Answer from the drawing. Dimensions are ordinates in mm from the lowest x, y and z of the part. Coordinates: 2 decimals unless noted, no trailing zeros. Order: outer loops, then holes, each group sorted by start corner. A loop starts at its lowest first (then second) coordinate and runs counter-clockwise, first axis right, second up. Notation, with made-up numbers: (83.5, 71) -> (105.5, 71) arc R18 cw to (105.5, 85) -> close; hole circle Ø2 at (-31.5, 79). An arc over 180 degrees is marked (long way). Answer as a JSON object with one key per item and string values. Group by question number.
1) Consider L1, parallel to Y at x = 95, z = 2.3; L2, parallel to X at y = 140, z = 3.25; L3, parallel to X at y = 130, z = 2.75. Determine where each line is inside the solid, lowest interval first.
2) Section A-A on z = 2.7 is taken. Determine the outline of the cut face in (x, y), and give its area (3 significant figures).
3) Section B-B on x = 60.5 is taken. Determine the outline of the cut face in (y, z), and give its area (3 significant figures).
4) Given pin 1 (2 mm diameter, centred on x = 68, z = 3.5, fed in from -Y); pin 2 (2 mm diameter, centred on y = 180, z = 3, fed in from -X), each flat-ended and moving along its own axis, determine where each tip first touches the part or whether it passes through.
5) Section C-C on y = 154 is taken. Determine the outline of the cut face in (x, z).
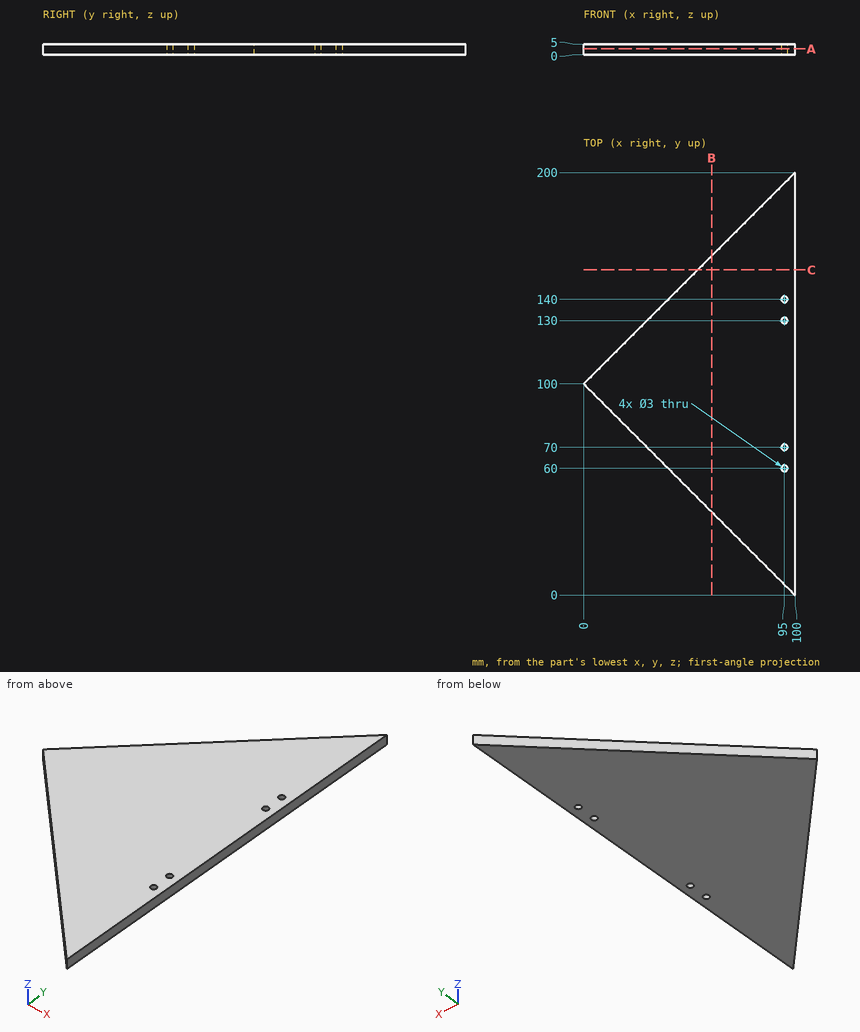
Worked answers:
{
 "1": {"L1": "y = 5 to 58.5, 61.5 to 68.5, 71.5 to 128.5, 131.5 to 138.5, 141.5 to 195", "L2": "x = 40 to 93.5, 96.5 to 100", "L3": "x = 30 to 93.5, 96.5 to 100"},
 "2": {"outline": "(0, 100) -> (100, 0) -> (100, 200) -> close; hole circle Ø3 at (95, 60); hole circle Ø3 at (95, 70); hole circle Ø3 at (95, 130); hole circle Ø3 at (95, 140)", "area": "9,970 mm²"},
 "3": {"outline": "(39.5, 0) -> (160.5, 0) -> (160.5, 5) -> (39.5, 5) -> close", "area": "605 mm²"},
 "4": {"pin 1": "stops at y = 31", "pin 2": "stops at x = 79"},
 "5": {"outline": "(54, 0) -> (100, 0) -> (100, 5) -> (54, 5) -> close"}
}
